The listing builds one solid part. Answer for the finished solid, in the listing's coordinates (mm). Round coordinates to 2 decimals unless told otherwise and drop trailing zeros. Write each loop counter-clockwise with the first axis right and the second up, starting at its lowest first coordinate (ties: lowest second). Pieces come first, ordered by that corner, then holes. Notation, with made-up numbers: (46.5, 55.5) - (79.5, 55.5) arc R14 ccw to (79.5, 73.5) - close; hole circle Ø7 at (52.25, -25.75). An arc over 180 degrees is marked (long way). Answer in a Markdown table with one row per item.
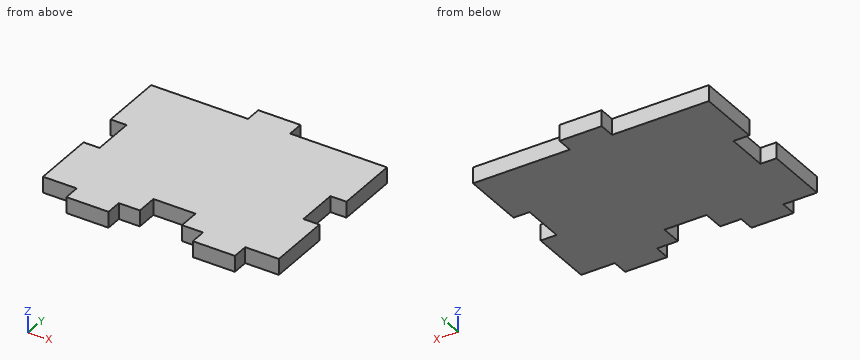
Autodesk Inventor part; units mm, degrees
ref_plane "YZ Plane" through (0, 0, 0) normal (1, 0, 0) x (0, 1, 0)
ref_plane "XZ Plane" through (0, 0, 0) normal (0, 1, 0) x (-1, 0, 0)
ref_plane "XY Plane" through (0, 0, 0) normal (0, 0, 1) x (1, 0, 0)
sketch "Sketch1" plane through (0, 0, 0) normal (0, 0, 1) x (1, 0, 0)
  line L0 (-38.1, 0) -> (38.1, 0)
  line L1 (38.1, 0) -> (38.1, 4.826)
  line L2 (-38.1, 4.826) -> (38.1, 4.826)
  line L3 (-38.1, 0) -> (-38.1, 4.826)
  line L4 (-25.4, 0) -> (-12.7, 0)
  line L5 (-25.4, 0) -> (-25.4, 4.826)
  line L6 (-12.7, 4.826) -> (-25.4, 4.826)
  line L7 (-12.7, 0) -> (-12.7, 4.826)
  line L8 (12.7, 0) -> (25.4, 0)
  line L9 (12.7, 0) -> (12.7, 4.826)
  line L10 (25.4, 4.826) -> (12.7, 4.826)
  line L11 (25.4, 0) -> (25.4, 4.826)
  point P0 (0, 0)
ref_plane "Work Plane1" through (-12.7, 0, -7.366) normal (0, 0, 1) x (1, 0, 0)
sketch "Sketch2" plane through (-12.7, 0, -7.366) normal (0, 0, 1) x (1, 0, 0)
  line L0 (0, 0) -> (-12.7, 0)
  line L1 (0, 0) -> (0, 4.826)
  line L2 (-12.7, 4.826) -> (0, 4.826)
  line L3 (-12.7, 0) -> (-12.7, 4.826)
  line L4 (-12.7, 0) -> (0, 0)
  line L5 (0, 0) -> (0, 4.826)
  line L6 (-12.7, 4.826) -> (-12.7, 0)
  line L7 (38.1, 0) -> (25.4, 0)
  line L8 (38.1, 0) -> (38.1, 4.826)
  line L9 (25.4, 4.826) -> (38.1, 4.826)
  line L10 (25.4, 0) -> (25.4, 4.826)
  line L11 (25.4, 0) -> (38.1, 0)
  line L12 (38.1, 0) -> (38.1, 4.826)
  line L13 (25.4, 4.826) -> (25.4, 0)
  line L14 (-18.034, 0) -> (-22.86, 0)
  line L15 (-18.034, 0) -> (-18.034, 4.826)
  line L16 (-22.86, 4.826) -> (-18.034, 4.826)
  line L17 (-22.86, 0) -> (-22.86, 4.826)
  line L18 (43.434, 0) -> (48.26, 0)
  line L19 (43.434, 0) -> (43.434, 4.826)
  line L20 (48.26, 4.826) -> (43.434, 4.826)
  line L21 (48.26, 0) -> (48.26, 4.826)
  line L22 (48.26, 55.626) -> (-22.86, 55.626)
  line L23 (-22.86, 36.576) -> (-18.034, 36.576)
  line L24 (-18.034, 36.576) -> (-18.034, 23.876)
  line L25 (-18.034, 23.876) -> (-22.86, 23.876)
  line L26 (48.26, 36.576) -> (43.434, 36.576)
  line L27 (43.434, 36.576) -> (43.434, 23.876)
  line L28 (43.434, 23.876) -> (48.26, 23.876)
  line L29 (-22.86, 55.626) -> (-22.86, 36.576)
  line L30 (-22.86, 23.876) -> (-22.86, 4.826)
  line L31 (48.26, 4.826) -> (48.26, 23.876)
  line L32 (48.26, 36.576) -> (48.26, 55.626)
  line L33 (-22.86, 4.826) -> (-12.7, 4.826)
  line L34 (0, 4.826) -> (25.4, 4.826)
  line L35 (38.1, 4.826) -> (48.26, 4.826)
  point P0 (12.7, 0)
  dimension "d0" = 50.8
  dimension "d2" = 12.7
  dimension "d5" = 4.826
  dimension "d18" = 19.05
  dimension "d19" = 19.05
extrude "Extrusion1" add sketch "Sketch2" along normal blind 4.826 contours L0 L3 L2 L1 | L2 L33 L16 L30 L25 L24 L23 L29 L22 L32 L26 L27 L28 L31 L20 L35 L9 L34 | L9 L8 L7 L10
sketch "Sketch3" plane through (-12.7, 0, -2.54) normal (0, 0, 1) x (1, 0, 0)
  line L0 (48.26, 55.626) -> (-22.86, 55.626)
  line L1 (-22.86, 55.626) -> (-22.86, 36.576)
  line L2 (48.26, 55.626) -> (-22.86, 55.626)
  line L3 (6.35, 55.626) -> (19.05, 55.626)
  line L4 (19.05, 55.626) -> (19.05, 60.452)
  line L5 (19.05, 60.452) -> (6.35, 60.452)
  line L6 (6.35, 60.452) -> (6.35, 55.626)
  point P0 (12.7, 0)
  dimension "d8" = 12.7
  dimension "d9" = 4.826
  dimension "d10" = 29.21
extrude "Extrusion2" add sketch "Sketch3" against normal blind 4.826
sketch "Sketch4" plane through (-12.7, 0, -2.54) normal (0, 0, 1) x (1, 0, 0)
  line L0 (0, 4.826) -> (25.4, 4.826)
  line L1 (6.35, 4.826) -> (19.05, 4.826)
  line L2 (19.05, 4.826) -> (19.05, 11.176)
  line L3 (19.05, 11.176) -> (6.35, 11.176)
  line L4 (6.35, 11.176) -> (6.35, 4.826)
  line L5 (48.26, 4.826) -> (48.26, 23.876)
  point P0 (12.7, 0)
  dimension "d13" = 12.7
  dimension "d14" = 6.35
  dimension "d15" = 29.21
extrude "Extrusion3" cut sketch "Sketch4" against normal blind 4.826
properties part number "sideR"
(1) Section D-D (y = 57) is taken. Give the vertices of the cut face in (x, z), and give its area (3 significant figures).
Checked values:
| item | result |
|---|---|
| outline | (-6.35, -7.37) - (6.35, -7.37) - (6.35, -2.54) - (-6.35, -2.54) - close |
| area | 61.3 mm2 |
(2) Flat-ended cylindrical pins translate along their axes: pin 1 (1.4 mm diameter, centred on x = -32, z = -5, fed in from +Y); pin 2 (2.5 mm diameter, centred on x = 34.5, z = -5, fed in from -Y); pin 3 (1.5 mm diameter, centred on x = 5.5, z = -4.5, fed in from -Y). Find the tip coordinate at first contact, or state that the pin passes through.
Checked values:
| item | result |
|---|---|
| pin 1 | stops at y = 55.63 |
| pin 2 | stops at y = 4.83 |
| pin 3 | stops at y = 11.18 |
(3) Section C-C (x = -2.5) is taken. Give the vertices of the cut face in (y, z).
Checked values:
| item | result |
|---|---|
| outline | (11.18, -7.37) - (60.45, -7.37) - (60.45, -2.54) - (11.18, -2.54) - close |
(4) Section A-A (y = 8.5) is taken. Give the vertices of the cut face in (x, z), and give its area (3 significant figures).
Checked values:
| item | result |
|---|---|
| outline | (-35.56, -7.37) - (-6.35, -7.37) - (-6.35, -2.54) - (-35.56, -2.54) - close; (6.35, -7.37) - (35.56, -7.37) - (35.56, -2.54) - (6.35, -2.54) - close |
| area | 282 mm2 |
(5) Section B-B (z = -4.3) is taken. Give the vertices of the cut face in (x, y).
Checked values:
| item | result |
|---|---|
| outline | (-35.56, 4.83) - (-25.4, 4.83) - (-25.4, 0) - (-12.7, 0) - (-12.7, 4.83) - (-6.35, 4.83) - (-6.35, 11.18) - (6.35, 11.18) - (6.35, 4.83) - (12.7, 4.83) - (12.7, 0) - (25.4, 0) - (25.4, 4.83) - (35.56, 4.83) - (35.56, 23.88) - (30.73, 23.88) - (30.73, 36.58) - (35.56, 36.58) - (35.56, 55.63) - (6.35, 55.63) - (6.35, 60.45) - (-6.35, 60.45) - (-6.35, 55.63) - (-35.56, 55.63) - (-35.56, 36.58) - (-30.73, 36.58) - (-30.73, 23.88) - (-35.56, 23.88) - close |
(6) Find the intervals of material crossed by line 1 (X direction, y = 24.5, z = -4.4); line 2 (Y direction, x = 27, z = -6.1); line 3 (Y direction, x = 22.5, z = -4.35), in increasing order.
Checked values:
| item | result |
|---|---|
| line 1 | x = -30.73 to 30.73 |
| line 2 | y = 4.83 to 55.63 |
| line 3 | y = 0 to 55.63 |
